Could you check a few things on this model? Use its own coordinates, in mm. Face numbers are marked on the shaded views. Coordinates: 2 decimals unless noted, no trailing zeros. Write each loop counter-clockwise with the first axis right and the second up, starting at its lowest first coordinate (ties: lowest second). Pieces come first, ordered by that corner, then holes. Notation, with made-up numbers: (47.25, 72) - (76.25, 72) arc R21 ccw to (76.25, 94) - close; hole circle Ø7 at (3, -18). An arc over 180 degrees is marked (long way). Answer as a JSON object with one key per item and string values. Group by question number.
1) If we section it at A-A (y = -37): Write out the boundary of the cut face in (x, z).
2) We'd pull the mould along Z, two halves only. Please class the marked faces 1, 2, 3 and 4: released by +Z, released by -Z, zero draft, split by the parting line, or undercut.
3) If we section it at D-D (x = 3.3): Write out the boundary of the cut face in (y, z).
4) Please list where these lines run through material, in increasing order: line 1 along Z through (x, y) = (2.85, -26.5); line 2 along Z through (x, y) = (2.9, -21); line 3 along Y through (x, z) = (4.25, 4.5).
5) If we section it at B-B (z = -13): Write out the boundary of the cut face in (x, y), plus the area to 3 significant figures.
6) If we section it at C-C (y = -8.5): Write out the boundary of the cut face in (x, z), plus the area to 3 significant figures.
7) Will these pins go through, and if not, where does the flat tip stop? pin 1 Ø1.8 at (x, y) = (3.5, -25) entering from +Z; pin 2 Ø3 at (x, z) = (3.5, 7) entering from -Y; pin 3 Ø1.8 at (x, z) = (1.5, 45.5) entering from +Y; pin 4 Ø9 at (y, z) = (-5.26, -15.83) entering from +X.
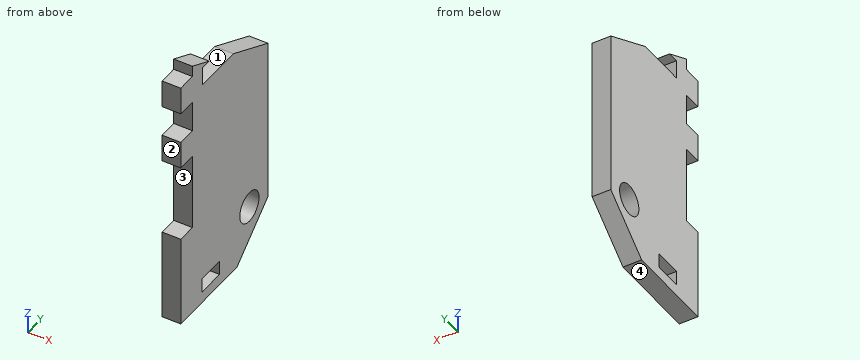
```python
from build123d import *

# Parameters (mm, degrees)
SKETCH1_W           = 4.681910348
SKETCH1_H           = 9.021241889
SKETCH1_R           = 5
BOSS_EXTRUDE1_DEPTH = 6


with BuildPart() as part:
    # Sketch1 → Boss-Extrude1 (new body)
    with BuildSketch(Plane(origin=(0, 0, 0), x_dir=(0, 0, -1), z_dir=(1, 0, 0))):
        Polygon((-49.613790305, -26.17980707), (-53.776961548, -34.881370998), (-50.167110133, -34.881370998), (-50.167110133, -40.881370998), (-41.167110133, -40.881370998), (-41.167110133, -34.881370998), (-31.167110133, -34.881370998), (-31.167110133, -40.881370998), (-22.167110133, -40.881370998), (-22.167110133, -34.881370998), (2.832889867, -34.881370998), (2.832889867, -40.881370998), (32.552897546, -40.881370998), (32.552897546, -11.700957806), (18.820856333, 4.303972987), (-35.029148102, 4.303972987), (-43.613790305, -13.639034538), (-43.613790305, -29.701183485), (-49.613790305, -29.701183485), align=None)
        with Locations((26.557768442, -25.304755476)):
            Rectangle(SKETCH1_W, SKETCH1_H, mode=Mode.SUBTRACT)
        with Locations((15.832889867, -5.263895329)):
            Circle(SKETCH1_R, mode=Mode.SUBTRACT)
    extrude(amount=BOSS_EXTRUDE1_DEPTH)


solid = part.part
```
Here are the results:
{
 "1": {"outline": "(0, -32.55) - (6, -32.55) - (6, -2.83) - (0, -2.83) - close; (0, 22.17) - (6, 22.17) - (6, 31.17) - (0, 31.17) - close; (0, 41.17) - (6, 41.17) - (6, 50.17) - (0, 50.17) - close"},
 "2": {"face 1": "undercut", "face 2": "zero draft", "face 3": "undercut", "face 4": "released by -Z"},
 "3": {"outline": "(-40.88, -32.55) - (-11.7, -32.55) - (4.3, -18.82) - (4.3, 35.03) - (-13.64, 43.61) - (-29.7, 43.61) - (-29.7, 49.61) - (-26.18, 49.61) - (-34.88, 53.78) - (-34.88, 50.17) - (-40.88, 50.17) - (-40.88, 41.17) - (-34.88, 41.17) - (-34.88, 31.17) - (-40.88, 31.17) - (-40.88, 22.17) - (-34.88, 22.17) - (-34.88, -2.83) - (-40.88, -2.83) - close; hole (-29.82, -28.9) - (-20.79, -28.9) - (-20.79, -24.22) - (-29.82, -24.22) - close; hole circle Ø10 at (-5.26, -15.83)"},
 "4": {"line 1": "z = -32.55 to -28.9, -24.22 to 43.61, 49.61 to 49.77", "line 2": "z = -32.55 to -28.9, -24.22 to 43.61", "line 3": "y = -34.88 to 4.3"},
 "5": {"outline": "(0, -40.88) - (6, -40.88) - (6, -9.38) - (0, -9.38) - close; (0, -1.14) - (6, -1.14) - (6, 4.3) - (0, 4.3) - close", "area": "222 mm²"},
 "6": {"outline": "(0, -29.81) - (6, -29.81) - (6, -19.64) - (0, -19.64) - close; (0, -12.02) - (6, -12.02) - (6, 41.16) - (0, 41.16) - close", "area": "380 mm²"},
 "7": {"pin 1": "stops at z = 43.61", "pin 2": "stops at y = -34.88", "pin 3": "stops at y = -29.7", "pin 4": "passes through"}
}
